from build123d import *

# Parameters (mm, degrees)
F0_W     = 134.382621
F0_H     = 86.09888
F1_DEPTH = 76.2
F2_W     = 121.511206
F2_H     = 74.4575
F3_DEPTH = 61.468
F4_R     = 5.454336
F4_R_2   = 6.504008
F5_DEPTH = 177.8


with BuildPart() as f1:
    # F0 (on Front) → F1 (new body)
    with BuildSketch(Plane.XZ):
        with Locations((0.213645, -2.778597)):
            Rectangle(F0_W, F0_H)
    extrude(amount=-F1_DEPTH)

    # F2 (on face) → F3 (cut)
    with BuildSketch(Plane.XZ):
        with Locations((-0.984143, -3.911963)):
            Rectangle(F2_W, F2_H)
    extrude(amount=-F3_DEPTH, mode=Mode.SUBTRACT)

    # F4 (on face) → F5 (cut)
    with BuildSketch(Plane.XY.offset(40.270843)):
        with Locations((-52.633329, 6.413179)):
            Circle(F4_R)
        with Locations((52.010948, 7.588945)):
            Circle(F4_R_2)
    extrude(amount=-F5_DEPTH, mode=Mode.SUBTRACT)


solid = f1.part
Can you work these out from the model? Positions are in its coordinate system, mm. A direction names the side the tool comes from. Give positions to 0.01 mm unless a question says otherwise; leave off trailing zeros. Order: outer loops, then holes, each group sorted by start corner. A loop starts at its lowest first (then second) coordinate and runs counter-clockwise, first axis right, second up. Notation, with made-up numbers: M 42.25,46.5 L 69.25,46.5 A5 ccw 69.25,50.5 Z; hole C 46,74 d9. An arc over 180 degrees is marked long. One line per question, with ' | ' between items.
Item 1: Please list where these lines run through material, in increasing order: L1, parallel to Z at x = 7.5, y = 14.5; L2, parallel to X at y = 7.5, z = -6; L3, parallel to Y at x = -51, z = -1.5.
Answer block:
L1: z = -45.83 to -41.14, 33.32 to 40.27 | L2: x = -66.98 to -61.74, 59.77 to 67.4 | L3: y = 61.47 to 76.2
Item 2: Suppose I cut it at B-B, the plane z = 22. Write out the boundary of the cut face in (x, y), then the cut area to 3 significant figures.
Answer block:
outline: M -66.98,0 L -61.74,0 L -61.74,61.47 L 59.77,61.47 L 59.77,0 L 67.4,0 L 67.4,76.2 L -66.98,76.2 Z | area: 2,770 mm2
Item 3: We'd pull the mould along X, two halves only. Please class faces 1 (the face through (-58.082, 6.653, 36.842)), 2 (the face through (0, 0, 36)), 3 (the face through (67.405, 38, -3)), 4 (the face through (59.771, 30, -4)): released by +X, released by -X, zero draft, split by the parting line, or undercut.
Answer block:
face 1: undercut | face 2: zero draft | face 3: released by +X | face 4: undercut
Item 4: Suppose I cut it at C-C, the plane x = -41. Write out the boundary of the cut face in (y, z), then the cut area to 3 significant figures.
Answer block:
outline: M 0,-45.83 L 76.2,-45.83 L 76.2,40.27 L 0,40.27 L 0,33.32 L 61.47,33.32 L 61.47,-41.14 L 0,-41.14 Z | area: 1,980 mm2
Item 5: Suppose I cut it at A-A, the plane y = 58. Write out the boundary of the cut face in (x, z), then the cut area to 3 significant figures.
Answer block:
outline: M -66.98,-45.83 L 67.4,-45.83 L 67.4,40.27 L -66.98,40.27 Z; hole M -61.74,-41.14 L 59.77,-41.14 L 59.77,33.32 L -61.74,33.32 Z | area: 2,520 mm2
Item 6: I'm going to push a flat-ended pin straight in: pin 1 Ø8 at (x, z) = (4.5, -37) entering from -Y. Where does the tip first touch, or does it pass through?
Answer block:
pin 1: stops at y = 61.47
Item 7: For faces 5 (the face through (-2, 30, 33.317)), 6 (the face through (58.215, 9.543, -43.452)), which set-ups out of +Z, -Z, +X, -X, +Y, -Y let a thin tool reach every point of the face, with its end or its side?
Answer block:
face 5: -Y | face 6: +Z, -Z
